Read the model definition and answer for the solid it produces. Units are mm, in the model's axes. Face numbers are marked on the shaded views. A direction names the side the tool comes from. Coordinates: 2 decimals unless noted, no trailing zeros. Write each loop counter-clockwise with the first axis right and the second up, starting at its lowest first coordinate (ties: lowest second). Pieces come first, ordered by that corner, then holes. Notation, with made-up numbers: (32.5, 20.5) -> (81.5, 20.5) arc R18 cw to (81.5, 36.5) -> close; hole circle Ø3 at (27.25, 12). An arc over 180 degrees is marked (long way). Write item = value, one per line. Start each with the question number.
1) Flat-ended cylindrical pins translate along their axes: pin 1 Ø3.5 at (x, z) = (5, 5.5) entering from +Y; pin 2 Ø8 at (x, z) = (1.5, 4) entering from -Y; pin 3 Ø4 at (x, z) = (6.5, 14.5) entering from -Y. Find the tip coordinate at first contact, or state that the pin passes through.
2) Section D-D (z = 10.5) is taken. Determine the outline of the cut face in (x, y).
3) A tool of negligible diameter and unlimited length cuts with its end or side. For the marked faces 1, 2, 3 and 4, from which of +Z, -Z, +X, -X, +Y, -Y can it reach the whole face along a straight path? Write none if from no direction.
4) Section C-C (x = -6) is taken. Determine the outline of the cut face in (y, z), plus the area to 3 significant figures.
5) Section B-B (y = -6) is taken. Determine the outline of the cut face in (x, z).
6) Find the intervals of material crossed by line 1 along X through (y, z) = (-4, 13.25); line 2 along Y through (x, z) = (7.75, 15); line 3 along Y through (x, z) = (5.75, 8.5), in increasing order. Write a range as from..to.
7) Section A-A (z = 5) is taken. Determine the outline of the cut face in (x, y).
8) For a pull along Z with two mould halves and no side action, classify the marked faces 5, 6 and 7 as released by +Z, released by -Z, zero draft, split by the parting line, or undercut.
from build123d import *

# Parameters (mm, degrees)
EXTRUDE_1_DEPTH     = 20
FILLET_1_R          = 10
SKETCH_2_R          = 2.1
CUT_EXTRUDE_1_DEPTH = 40.195025195


with BuildPart() as part:
    # 草图1 → 凸台-拉伸1 (new body)
    with BuildSketch(Plane.XY):
        Polygon((3.3, 0), (10, 0), (10, -17), (0, -17), (-5, -17), (-5, -28.5), (-8, -28.5), (-8, 11.5), (-5, 11.5), (-5, 0), (0, 0), (0, -12), (3.3, -12), align=None)
    extrude(amount=EXTRUDE_1_DEPTH)

    # 圆角1
    # the kernel refuses this fillet: 10 mm, written as the material it adds along each edge
    with BuildSketch(Plane(origin=(-5, -17, 0), x_dir=(0, -1, 0), z_dir=(0, 0, 1))) as fillet_1_piece_1:
        with BuildLine():
            CenterArc((FILLET_1_R, FILLET_1_R), FILLET_1_R, 180, 90)
            Line((0, FILLET_1_R), (-FILLET_1_R * 0.02, FILLET_1_R))
            Line((-FILLET_1_R * 0.02, FILLET_1_R), (-FILLET_1_R * 0.02, -FILLET_1_R * 0.02))
            Line((-FILLET_1_R * 0.02, -FILLET_1_R * 0.02), (FILLET_1_R, -FILLET_1_R * 0.02))
            Line((FILLET_1_R, -FILLET_1_R * 0.02), (FILLET_1_R, 0))
        make_face()
    extrude(amount=20)
    with BuildSketch(Plane(origin=(-5, 0, 0), x_dir=(1, 0, 0), z_dir=(0, 0, 1))) as fillet_1_piece_2:
        with BuildLine():
            CenterArc((10, 8.660254038), FILLET_1_R, 180, 60)
            Line((0, 8.660254038), (-0.2, 8.660254038))
            Line((-0.2, 8.660254038), (-0.2, 0))
            Line((-0.2, 0), (0, -0.2))
            ThreePointArc((0, -0.2), (2.5, -0.2), (4.9, -0.173205081))
            Line((4.9, -0.173205081), (5, 0))
        make_face()
    extrude(amount=20)

    # 草图2 → 切除-拉伸1 (cut, through all)
    with BuildSketch(Plane.ZY.offset(8)):
        with Locations((5, -6)):
            Circle(SKETCH_2_R)
        with Locations((15, -6)):
            Circle(SKETCH_2_R)
    extrude(amount=-CUT_EXTRUDE_1_DEPTH, mode=Mode.SUBTRACT)


solid = part.part
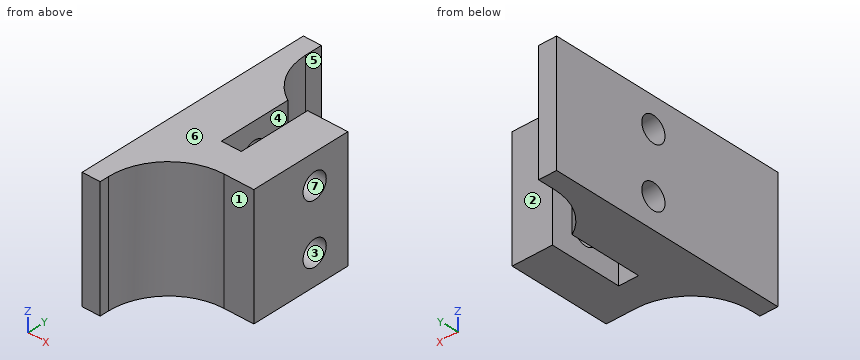
Answer key:
q1.pin_1 = 0
q1.pin_2 = -20.39
q1.pin_3 = -17.01
q2.outline = (-8, -28.5) -> (-5, -28.5) -> (-5, -27) arc R10 cw to (5, -17) -> (10, -17) -> (10, 0) -> (3.3, 0) -> (3.3, -12) -> (0, -12) -> (0, 0) arc R10 cw to (-5, 8.66) -> (-5, 11.5) -> (-8, 11.5) -> close
q3.face_1 = +Z, -Z, +X, -Y
q3.face_2 = +Z, -Z, +X, +Y
q3.face_3 = +X, -X
q3.face_4 = +Z, -Z, +Y
q4.outline = (-28.5, 0) -> (11.5, 0) -> (11.5, 20) -> (-28.5, 20) -> close; hole circle Ø4.2 at (-6, 5); hole circle Ø4.2 at (-6, 15)
q4.area = 772 mm^2
q5.outline = (-8, 0) -> (0, 0) -> (0, 2.9) -> (-8, 2.9) -> close; (-8, 7.1) -> (0, 7.1) -> (0, 12.9) -> (-8, 12.9) -> close; (-8, 17.1) -> (0, 17.1) -> (0, 20) -> (-8, 20) -> close; (3.3, 0) -> (10, 0) -> (10, 2.9) -> (3.3, 2.9) -> close; (3.3, 7.1) -> (10, 7.1) -> (10, 12.9) -> (3.3, 12.9) -> close; (3.3, 17.1) -> (10, 17.1) -> (10, 20) -> (3.3, 20) -> close
q6.line_1 = -8..0, 3.3..10
q6.line_2 = -17..-8.1, -3.9..0
q6.line_3 = -17..0
q7.outline = (-8, -28.5) -> (-5, -28.5) -> (-5, -27) arc R10 cw to (5, -17) -> (10, -17) -> (10, -8.1) -> (3.3, -8.1) -> (3.3, -12) -> (0, -12) -> (0, -8.1) -> (-8, -8.1) -> close; (-8, -3.9) -> (0, -3.9) -> (0, 0) arc R10 cw to (-5, 8.66) -> (-5, 11.5) -> (-8, 11.5) -> close; (3.3, -3.9) -> (10, -3.9) -> (10, 0) -> (3.3, 0) -> close
q8.face_5 = zero draft
q8.face_6 = released by +Z
q8.face_7 = undercut
